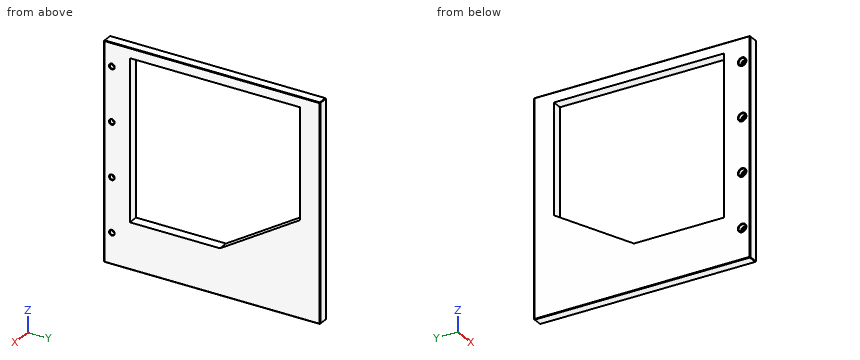
from build123d import *

# Parameters (mm, degrees)
SKETCH011_W     = 216
SKETCH011_H     = 216
PAD005_DEPTH    = 10
SKETCH014_R     = 2.35
POCKET008_DEPTH = 11
SKETCH015_R     = 3.75
POCKET009_DEPTH = 5
CHAMFER001_SIZE = 0.5
POCKET010_DEPTH = 10


with BuildPart() as part:
    # Sketch011 → Pad005 (new body)
    with BuildSketch(Plane.YZ):
        with Locations((92, -108)):
            Rectangle(SKETCH011_W, SKETCH011_H)
    extrude(amount=-PAD005_DEPTH)

    # Sketch014 (on Face6 of Pad005) → Pocket008 (cut)
    with BuildSketch(Plane(origin=(-10, 0, 0), x_dir=(0, 1, 0), z_dir=(-1, 0, 0))):
        with Locations((-8.060639, 185.203074)):
            Circle(SKETCH014_R)
        with Locations((-8.060639, 131.203074)):
            Circle(SKETCH014_R)
        with Locations((-8.060639, 77.203074)):
            Circle(SKETCH014_R)
        with Locations((-8.060639, 23.203074)):
            Circle(SKETCH014_R)
    extrude(amount=-POCKET008_DEPTH, mode=Mode.SUBTRACT)

    # Sketch015 (on Face5 of Pocket008) → Pocket009 (cut)
    with BuildSketch(Plane(origin=(-10, 0, 0), x_dir=(0, 1, 0), z_dir=(-1, 0, 0))):
        with Locations((-8.071904, 23.147722)):
            Circle(SKETCH015_R)
        with Locations((-8.071904, 77.147722)):
            Circle(SKETCH015_R)
        with Locations((-8.071904, 131.147722)):
            Circle(SKETCH015_R)
        with Locations((-8.071904, 185.147722)):
            Circle(SKETCH015_R)
    extrude(amount=-POCKET009_DEPTH, mode=Mode.SUBTRACT)

    # Chamfer001
    chamfer001_edges = [part.edges().sort_by_distance(p)[0] for p in [
        (-5, -16, 0),
        (-5, -16, -216),
        (0, -16, -108),
        (-10, -16, -108),
        (-5, 200, 0),
        (0, 92, 0),
        (-10, 92, 0),
        (-5, 200, -216),
        (0, 92, -216),
        (-10, 92, -216),
        (0, 200, -108),
        (0, -10.410639, -185.203074),
        (0, -10.410639, -131.203074),
        (0, -10.410639, -77.203074),
        (0, -10.410639, -23.203074),
        (-10, 200, -108),
        (-10, -11.821904, -23.147722),
        (-10, -11.821904, -185.147722),
        (-10, -11.821904, -131.147722),
        (-10, -11.821904, -77.147722),
        (-5, -10.410639, -185.203074),
        (-2.5, -5.710639, -185.203074),
        (-5, -10.410639, -131.203074),
        (-2.5, -5.710639, -131.203074),
        (-5, -10.410639, -77.203074),
        (-2.5, -5.710639, -77.203074),
        (-5, -10.410639, -23.203074),
        (-2.5, -5.710639, -23.203074),
        (-7.5, -4.321904, -23.147722),
        (-5, -11.821904, -23.147722),
        (-7.5, -4.321904, -185.147722),
        (-5, -11.821904, -185.147722),
        (-7.5, -4.321904, -131.147722),
        (-5, -11.821904, -131.147722),
        (-7.5, -4.321904, -77.147722),
        (-5, -11.821904, -77.147722),
    ]]
    chamfer(chamfer001_edges, length=CHAMFER001_SIZE)

    # Sketch016 (on Face11 of Chamfer001) → Pocket010 (cut)
    with BuildSketch(Plane(origin=(-10, 0, 0), x_dir=(0, 1, 0), z_dir=(-1, 0, 0))):
        Polygon((180, 10), (10, 10), (10, 170), (100, 170), (180, 120), align=None)
    extrude(amount=-POCKET010_DEPTH, mode=Mode.SUBTRACT)


solid = part.part
For this review, take the finished solid that the model builds, in its own axes (mm). Give positions to 0.01 mm unless a question says otherwise; leave off trailing zeros. Loops run counter-clockwise (first coordinate to the right, second up) from the corner with the lowest first, then second, coordinate; pieces in that order, holes last.
Item 1: For line 1 along Z through (x, y) = (-4.5, 62); line 2 along Y through (x, z) = (-5.75, -22.5); line 3 along Y through (x, z) = (-3.25, -25), list the stretches that pass through material, from the lowest coordinate up.
Item 2: Insertion check: pin 1 (1.5 mm diameter, centred on y = 14, z = -167.5, fed in from +X); pin 2 (5 mm diameter, centred on y = -8.5, z = -75.5, fed in from -X); pin 3 (5.5 mm diameter, centred on y = -8.06, z = -131.2, fed in from -X); pin 4 (3 mm diameter, centred on y = -6.5, z = -131.5, fed in from -X). Each pin has a flat end and moves straight along its axis. Give the tip position at first contact, or say it passes through.
Item 3: Take a section at C-C, the plane x = -2.75. State the section outline as (y, z) points, and give its area (3 significant figures).
Item 4: Take a section at B-B, the plane y = 81. State the section outline as (x, z) points.
Item 5: Take a section at A-A, the plane z = -107. State the section outline as (x, y) points, and give its area (4 significant figures).
Calculated:
1. line 1: z = -216 to -170, -10 to 0
1. line 2: y = -16 to -11.77, -4.38 to 10, 180 to 200
1. line 3: y = -16 to -9.58, -6.55 to 10, 180 to 200
2. pin 1: passes through
2. pin 2: stops at x = -9.95
2. pin 3: stops at x = -4.9
2. pin 4: stops at x = -5
3. outline: (-16, -215.5) - (-15.5, -216) - (199.5, -216) - (200, -215.5) - (200, -0.5) - (199.5, 0) - (-15.5, 0) - (-16, -0.5) - close; hole circle Ø4.7 at (-8.06, -185.2); hole circle Ø4.7 at (-8.06, -131.2); hole circle Ø4.7 at (-8.06, -77.2); hole circle Ø4.7 at (-8.06, -23.2); hole (10, -170) - (100, -170) - (180, -120) - (180, -10) - (10, -10) - close
3. area: 21,400 mm2
4. outline: (-10, -215.5) - (-9.5, -216) - (-0.5, -216) - (0, -215.5) - (0, -170) - (-10, -170) - close; (-10, -10) - (0, -10) - (0, -0.5) - (-0.5, 0) - (-9.5, 0) - (-10, -0.5) - close
5. outline: (-10, -15.5) - (-9.5, -16) - (-0.5, -16) - (0, -15.5) - (0, 10) - (-10, 10) - close; (-10, 180) - (0, 180) - (0, 199.5) - (-0.5, 200) - (-9.5, 200) - (-10, 199.5) - close
5. area: 459.5 mm2
